Verification items for the finished model (mm, model axes). A direction names the side the tool comes from. Coordinates: 2 decimals unless noted, no trailing zeros. Loops run counter-clockwise (first coordinate to the right, second up) from the corner with the lowest first, then second, coordinate; pieces in that order, holes last. Notation, with made-up numbers: (42.5, 60.5) -> (51.5, 60.5) arc R33 cw to (51.5, 96.5) -> close; hole circle Ø7 at (50, 62.5). An arc over 180 degrees is marked (long way). Answer as a JSON object with one key per item and string values. Group by question number.
Q1. Cross-section at C-C on y = -7. Record the boundary of the cut face in (x, z).
Q2. Scan lines: L1, parallel to Z at x = 3.5, y = -22; L2, parallel to Z at x = -34, y = -42.5; L3, parallel to X at y = -3.5, z = -1. Record each from-to range of solid material in increasing order.
Q3. Set-up check for faces 5 (the cylindrical face through (-12.698, -36.434, -61.158)), 6 (the flat face through (-5, -26, 38.727)), 7 (the flat face through (24, -41, 10.267)): record each of +Z, -Z, +X, -X, +Y, -Y from which the full face is reachable in a straight line by a thin tool's end or side.
Q4. Cross-section at B-B on z = 31.5. Record the boundary of the cut face in (x, y).
Q5. Gauge pin test, flat end, axial feed: pin 1 Ø7.5 at (x, z) = (-35.5, -1.5) entering from -Y. Record the tip position at first contact, or that the pin passes through.
Q6. Release check for a two-part mould opening along X. For faces 1 (the flat face through (-37.92, -25, -10)), 2 (the flat face through (-31.066, -26, -10)), 3 (the flat face through (21.17, -26, -10)), 4 (the flat face through (-6, -25, -63.982)) record: released by +X, released by -X, zero draft, split by the parting line, or undercut.
Q7. Cross-section at A-A on x = 11. Record the boundary of the cut face in (y, z), and give its area (3 significant figures).
Q8. Cross-section at D-D on x = -5. Record the boundary of the cut face in (y, z).
```python
from build123d import *

# Parameters (mm, degrees)
F0_W     = 64.112249
F0_H     = 108.938705
F1_DEPTH = 50.8
F3_W     = 52.236052
F3_H     = 96.981097
F4_DEPTH = 131.318
F2_W     = 19.592841
F2_H     = 38.154388
F5_DEPTH = 116.078
F6_R     = 6.513385
F7_DEPTH = 143.51


with BuildPart() as f1:
    # F0 (on Front) → F1 (new body)
    with BuildSketch(Plane.XZ):
        with Locations((-5.863925, -9.51259)):
            Rectangle(F0_W, F0_H)
    extrude(amount=F1_DEPTH)

    # F3 (on face) → F4 (cut)
    with BuildSketch(Plane.XZ.offset(50.8)):
        with Locations((-4.947773, -9.76373)):
            Rectangle(F3_W, F3_H)
    extrude(amount=-F4_DEPTH, mode=Mode.SUBTRACT)

    # F2 (on face) → F5 (cut)
    with BuildSketch(Plane(origin=(-37.92005, 0, 0), x_dir=(0, -1, 0), z_dir=(-1, 0, 0))):
        with Locations((41.00358, -8.810162)):
            Rectangle(F2_W, F2_H)
    extrude(amount=-F5_DEPTH, mode=Mode.SUBTRACT)

    # F6 (on face) → F7 (cut)
    with BuildSketch(Plane(origin=(0, 0, -63.981943), x_dir=(1, 0, 0), z_dir=(0, 0, -1))):
        with Locations((-7.528701, 40.396869)):
            Circle(F6_R)
    extrude(amount=-F7_DEPTH, mode=Mode.SUBTRACT)


solid = f1.part
```
Computed values:
{
 "1": {"outline": "(-37.92, -63.98) -> (26.19, -63.98) -> (26.19, 44.96) -> (-37.92, 44.96) -> close; hole (-31.07, -58.25) -> (21.17, -58.25) -> (21.17, 38.73) -> (-31.07, 38.73) -> close"},
 "2": {"L1": "z = -63.98 to -58.25, 38.73 to 44.96", "L2": "z = -63.98 to -27.89, 10.27 to 44.96", "L3": "x = -37.92 to -31.07, 21.17 to 26.19"},
 "3": {"face 5": "+Z, -Z", "face 6": "+Y, -Y", "face 7": "+X, -X, -Y"},
 "4": {"outline": "(-37.92, -50.8) -> (-31.07, -50.8) -> (-31.07, 0) -> (-37.92, 0) -> close; (21.17, -50.8) -> (26.19, -50.8) -> (26.19, 0) -> (21.17, 0) -> close"},
 "5": {"pin 1": "stops at y = -31.21"},
 "6": {"face 1": "released by -X", "face 2": "undercut", "face 3": "undercut", "face 4": "zero draft"},
 "7": {"outline": "(-50.8, -63.98) -> (0, -63.98) -> (0, -58.25) -> (-50.8, -58.25) -> close; (-50.8, 38.73) -> (0, 38.73) -> (0, 44.96) -> (-50.8, 44.96) -> close", "area": "607 mm²"},
 "8": {"outline": "(-50.8, -63.98) -> (-46.4, -63.98) -> (-46.4, -58.25) -> (-50.8, -58.25) -> close; (-50.8, 38.73) -> (-46.4, 38.73) -> (-46.4, 44.96) -> (-50.8, 44.96) -> close; (-34.39, -63.98) -> (0, -63.98) -> (0, -58.25) -> (-34.39, -58.25) -> close; (-34.39, 38.73) -> (0, 38.73) -> (0, 44.96) -> (-34.39, 44.96) -> close"}
}
